Here's how the part is built. I have some questions about the finished solid (model axes, mm). Face numbers are marked on the shaded views. A direction names the side the tool comes from. Coordinates: 2 decimals unless noted, no trailing zeros. Order: outer loops, then holes, each group sorted by start corner. A loop starts at its lowest first (then second) coordinate and runs counter-clockwise, first axis right, second up. Notation, with made-up numbers: (-18.5, -39.75) - (-14.5, -39.75) arc R15 cw to (-14.5, -31.75) - close; hole circle Ø10 at (7, 45). An arc over 180 degrees is marked (long way). Answer as CSV lines item,"result". Start each with the question number.
Item 1: Imagine slicing it at B-B on x = 5. Count the separate pieces of the cut face and the enclosed holes in it, and give its area (3 significant figures).
Item 2: Imagine slicing it at A-A on y = 28.5. List the corners of the cut face in (x, z) for me.
Item 3: On a 3-axis mill with a long thin cutter (end or side, diameter ignored), from which of +Z, -Z, +X, -X, +Y, -Y can I reach the whole of each face in a straight line? I mean the marked faces 1, 2 and 3. Say none if no direction works.
Item 4: I'm going to push flat-ended pins straight in: pin 1 (1 mm diameter, centred on x = 3.5, z = -75, fed in from +Y); pin 2 (2.5 mm diameter, centred on y = 37.1, z = -36.57, fed in from -X); pin 3 (1.8 mm diameter, centred on x = 4.5, z = -72, fed in from -Y). Where does each tip first touch, or does it pass through?
Item 5: I need wall thicknesses on line 1 (Z direction, x = 3.9, y = 42.5); line 2 (Y direction, x = 1.25, z = -36.5); line 3 (Y direction, x = 5.45, z = -27). Which ranges of each line are inside material? Lowest first, please.
Item 6: Imagine slicing it at C-C on y = 12.5. List the corners of the cut face in (x, z) for me, and give its area (3 significant figures).
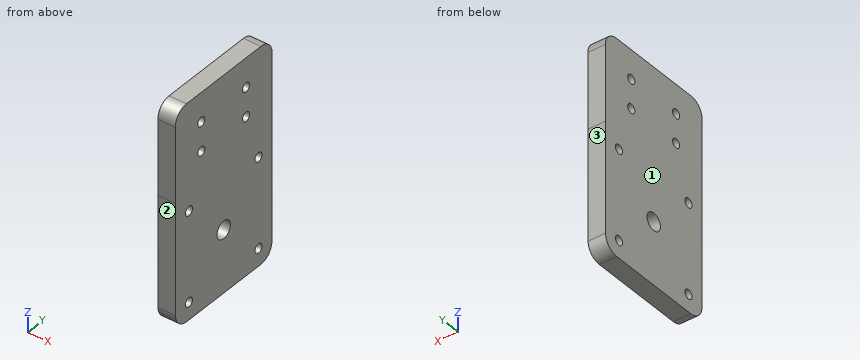
from build123d import *

# Parameters (mm, degrees)
F0_R     = 1.6
F0_R_2   = 3
F1_DEPTH = 6


with BuildPart() as f1:
    # F0 (on Right) → F1 (new body)
    with BuildSketch(Plane.YZ):
        with BuildLine():
            Line((5.599948, -47.575754), (5.599948, -85.56769))
            ThreePointArc((5.599948, -85.56769), (7.064414, -89.103224), (10.599948, -90.56769))
            Line((10.599948, -90.56769), (43.599948, -90.56769))
            ThreePointArc((43.599948, -90.56769), (47.135482, -89.103224), (48.599948, -85.56769))
            Line((48.599948, -85.56769), (48.599948, -47.575754))
            ThreePointArc((48.599948, -47.575754), (48.599955, -47.567689), (48.599974, -47.559625))
            Line((48.599974, -47.559625), (48.683767, -21.583819))
            ThreePointArc((48.683767, -21.583819), (47.225025, -18.037863), (43.683793, -16.56769))
            Line((43.683793, -16.56769), (10.516103, -16.56769))
            ThreePointArc((10.516103, -16.56769), (6.974871, -18.037863), (5.516129, -21.583819))
            Line((5.516129, -21.583819), (5.599922, -47.559625))
            ThreePointArc((5.599922, -47.559625), (5.599941, -47.567689), (5.599948, -47.575754))
        make_face()
        with Locations((11.599948, -84.56769)):
            Circle(F0_R, mode=Mode.SUBTRACT)
        with Locations((42.599948, -84.56769)):
            Circle(F0_R, mode=Mode.SUBTRACT)
        with Locations((27.099948, -69.06769)):
            Circle(F0_R_2, mode=Mode.SUBTRACT)
        with Locations((11.599948, -53.56769)):
            Circle(F0_R, mode=Mode.SUBTRACT)
        with Locations((17.099948, -36.56769)):
            Circle(F0_R, mode=Mode.SUBTRACT)
        with Locations((17.099948, -26.56769)):
            Circle(F0_R, mode=Mode.SUBTRACT)
        with Locations((37.099948, -36.56769)):
            Circle(F0_R, mode=Mode.SUBTRACT)
        with Locations((42.599948, -53.56769)):
            Circle(F0_R, mode=Mode.SUBTRACT)
        with Locations((37.099948, -26.56769)):
            Circle(F0_R, mode=Mode.SUBTRACT)
    extrude(amount=F1_DEPTH)


solid = f1.part
Responses:
1,separate pieces,"1"
1,enclosed holes,"9"
1,area,"3,070 mm^2"
2,outline,"(0, -90.57) - (6, -90.57) - (6, -71.72) - (0, -71.72) - close; (0, -66.41) - (6, -66.41) - (6, -16.57) - (0, -16.57) - close"
3,face 1,"+Z, -Z, -X, +Y, -Y"
3,face 2,"-Z, +X, -X, -Y"
3,face 3,"-Z, +X, -X, +Y"
4,pin 1,"stops at y = 48.6"
4,pin 2,"passes through"
4,pin 3,"stops at y = 5.6"
5,line 1,"z = -90.57 to -86.16, -82.97 to -55.16, -51.97 to -16.57"
5,line 2,"y = 5.56 to 15.5, 18.7 to 35.5, 38.7 to 48.64"
5,line 3,"y = 5.53 to 15.56, 18.64 to 35.56, 38.64 to 48.67"
6,outline,"(0, -90.57) - (6, -90.57) - (6, -85.89) - (0, -85.89) - close; (0, -83.24) - (6, -83.24) - (6, -54.89) - (0, -54.89) - close; (0, -52.24) - (6, -52.24) - (6, -16.57) - (0, -16.57) - close"
6,area,"412 mm^2"
